The model under review builds one solid part; all positions refer to its coordinate system, in mm. Face numbers are marked on the shaded views. A direction names the side the tool comes from. Round coordinates to 2 decimals unless told otherwise and drop trailing zeros. Loops run counter-clockwise (first coordinate to the right, second up) from the corner with the lowest first, then second, coordinate; pieces in that order, holes last. Notation, with made-up numbers: (-13.75, 36) -> (-7.75, 36) arc R10 ccw to (-7.75, 54) -> close; hole circle Ø4 at (39, 50). An arc over 180 degrees is marked (long way). Return JSON: item names as keys, results as strings. Group by question number.
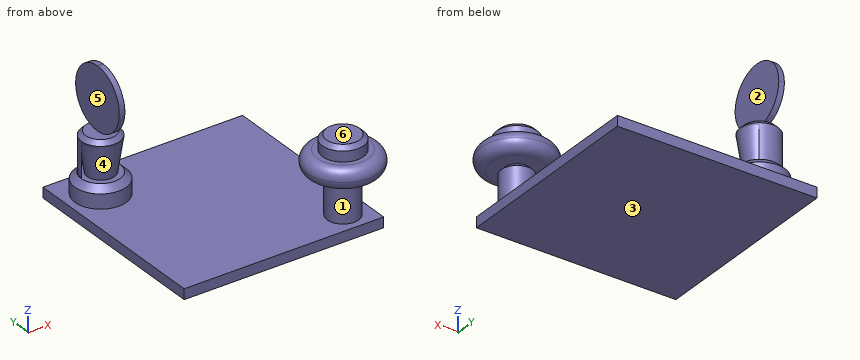
```python
from build123d import *

# Parameters (mm, degrees)
F0_W      = 97
F0_H      = 5
F1_DEPTH  = 48.5
F2_R      = 7.6458649313
F3_DEPTH  = 20
F4_SIZE   = 2
F5_R      = 17.4861306414
F6_DEPTH  = 10
F7_R      = 4.99999
F8_R      = 10
F9_DEPTH  = 7
F10_SIZE  = 2
F11_R     = 12.5
F12_DEPTH = 10
F13_SIZE  = 3
F14_R     = 9.2774942081
F15_DEPTH = 19
F16_SIZE  = 2
F17_W     = 2.7091787755
F17_H     = 30.5535356402
F18_DEPTH = 30
F20_DEPTH = 17.3555893878


# Not quite as in the source:
# - a fillet or chamfer is up to 0.001 mm smaller than in the source, because OpenCascade refuses the exact size


with BuildPart() as f1:
    # F0 (on Front) → F1 (new body, symmetric)
    with BuildSketch(Plane.XZ):
        with Locations((1.2960880995, -0.2472623394)):
            Rectangle(F0_W, F0_H)
    extrude(amount=F1_DEPTH, both=True)

    # F2 (on face) → F3 (join)
    with BuildSketch(Plane.XY.offset(2.2527376606)):
        with Locations((37.7960880995, -37.5)):
            Circle(F2_R)
    extrude(amount=F3_DEPTH)

    # F4
    f4_edges = [f1.edges().sort_by_distance(p)[0] for p in [
        (30.150223, -37.5, 22.252738),
    ]]
    chamfer(f4_edges, length=F4_SIZE)

    # F5 (on face) → F6 (join)
    with BuildSketch(Plane.XY.offset(22.2527376606)):
        with Locations((37.7960880995, -37.5)):
            Circle(F5_R)
    extrude(amount=F6_DEPTH)

    # F7 (radius 5 in the source; OpenCascade refuses exactly that, so slightly less here)
    f7_edges = [f1.edges().sort_by_distance(p)[0] for p in [
        (55.282219, -37.5, 27.252738),
        (20.309957, -37.5, 22.252738),
        (20.309957, -37.5, 32.252738),
    ]]
    fillet(f7_edges, radius=F7_R)

    # F8 (on face) → F9 (join)
    with BuildSketch(Plane.XY.offset(32.2527376606)):
        with Locations((37.7960880995, -37.5)):
            Circle(F8_R)
    extrude(amount=F9_DEPTH)

    # F10
    f10_edges = [f1.edges().sort_by_distance(p)[0] for p in [
        (27.796088, -37.5, 39.252738),
    ]]
    chamfer(f10_edges, length=F10_SIZE)

    # F11 (on face) → F12 (join)
    with BuildSketch(Plane.XY.offset(2.2527376606)):
        with Locations((-31.2039119005, 31.5)):
            Circle(F11_R)
    extrude(amount=F12_DEPTH)

    # F13
    f13_edges = [f1.edges().sort_by_distance(p)[0] for p in [
        (-43.703912, 31.5, 12.252738),
    ]]
    chamfer(f13_edges, length=F13_SIZE)

    # F14 (on face) → F15 (join)
    with BuildSketch(Plane.XY.offset(12.2527376606)):
        with Locations((-31.2039119005, 31.5)):
            Circle(F14_R)
    extrude(amount=F15_DEPTH)

    # F16
    f16_edges = [f1.edges().sort_by_distance(p)[0] for p in [
        (-40.481406, 31.5, 31.252738),
    ]]
    chamfer(f16_edges, length=F16_SIZE)

    # F17 (on face) → F18 (join)
    with BuildSketch(Plane.XY.offset(31.2527376606)):
        with Locations((-31.2039119005, 31.5)):
            Rectangle(F17_W, F17_H)
    extrude(amount=F18_DEPTH)

    # F19 (on face) → F20 (cut, through all)
    with BuildSketch(Plane.YZ.offset(-29.8493225127)):
        with BuildLine():
            Line((46.7767678201, 61.2527376606), (32.0485214627, 61.2527376606))
            ThreePointArc((32.0485214627, 61.2527376606), (42.4791618872, 56.763699091), (46.7767678201, 46.2527376606))
            Line((46.7767678201, 46.2527376606), (46.7767678201, 61.2527376606))
        make_face()
        with BuildLine():
            ThreePointArc((31.5, 31.2527376606), (16.7717536426, 46.2527376606), (31.5, 61.2527376606))
            Line((31.5, 61.2527376606), (16.2232321799, 61.2527376606))
            Line((16.2232321799, 61.2527376606), (16.2232321799, 31.2527376606))
            Line((16.2232321799, 31.2527376606), (24.3496846545, 31.2527376606))
            Line((24.3496846545, 31.2527376606), (31.5, 31.2527376606))
        make_face()
        with BuildLine():
            ThreePointArc((46.7767678201, 46.2527376606), (42.4791618872, 35.7417762302), (32.0485214627, 31.2527376606))
            Line((32.0485214627, 31.2527376606), (38.6503153455, 31.2527376606))
            Line((38.6503153455, 31.2527376606), (46.7767678201, 31.2527376606))
            Line((46.7767678201, 31.2527376606), (46.7767678201, 46.2527376606))
        make_face()
    extrude(amount=-F20_DEPTH, mode=Mode.SUBTRACT)

    # F22 (on offset) → F23 (revolve, cut)
    with BuildSketch(Plane.XZ.offset(-31.4)):
        Polygon((-21.9264176924, 12.2527376606), (-21.9264176924, 29.2527376606), (-24.4411546737, 12.2527376606), align=None)
        Polygon((-37.9155091941, 12.2527376606), (-40.4814061086, 29.2527376606), (-40.4814061086, 12.2527376606), align=None)
    revolve(axis=Axis((-31.1523377895, 31.4, 20.637573155), (0, 0, 1)), mode=Mode.SUBTRACT)


solid = f1.part
```
1. Wall thickness on line 1 (Z direction, x = 29, y = -44.5); line 2 (Z direction, x = -5, y = -6.5); line 3 (Y direction, x = 37.5, z = 5): over which ranges is each line inside the solid? List them lowest first.
2. Tool access review of the marked faces 4, 5 and 6: name each direction out of +Z, -Z, +X, -X, +Y, -Y from which nothing blocks a thin tool from reaching the whole face with its end or side.
3. We need section C-C, the plane y = 34. Give the number of separate pieces and of enclosed holes in the cut face, then the cut area to 3 significant figures.
4. Draft analysis for pull direction Z (two halves, no side actions). For the marked faces 1, 2 and 3, state which applies: pulls with the +Z half, pulls with the -Z half, needs draft (parallel to the pull), parting line crosses it, or undercut.
5. For P1, Ø3, axis at x = 44.5, z = 34, coming from the -Y side; P2, Ø8, axis at x = 36, y = -37.5, coming from the +Z side; P3, Ø2, axis at y = -28, z = 33.5, coming from the -X side, all flat-tipped, find the tip position at first contact; note any pin that passes through.
6. We need section D-D, the plane z = 35.5. Write out the cut boundary in (x, y).
7. We need section A-A, the plane z = 4. Write out the cut boundary in (x, y), then the cut area to 3 significant figures.
Check sheet entries:
{
 "1": {"line 1": "z = -2.75 to 2.25, 22.25 to 32.25", "line 2": "z = -2.75 to 2.25", "line 3": "y = -45.14 to -29.86"},
 "2": {"face 4": "none", "face 5": "+Z, -X, +Y, -Y", "face 6": "+Z, +X, -X, +Y, -Y"},
 "3": {"separate pieces": "2", "enclosed holes": "1", "area": "1,090 mm²"},
 "4": {"face 1": "undercut", "face 2": "needs draft", "face 3": "pulls with the -Z half"},
 "5": {"P1": "stops at y = -46.04", "P2": "stops at z = 39.25", "P3": "stops at x = 32.53"},
 "6": {"outline": "(-32.56, 21.31) -> (-29.85, 21.31) -> (-29.85, 42.24) -> (-32.56, 42.24) -> close; circle Ø20 at (37.8, -37.5)"},
 "7": {"outline": "circle Ø25 at (-31.2, 31.5); circle Ø15.29 at (37.8, -37.5)", "area": "675 mm²"}
}
